from build123d import *

# Parameters (mm, degrees)
F1_DEPTH = 11.75
F3_DEPTH = 10.2
F4_R     = 3
F5_DEPTH = 12.5
F6_R     = 0.5


with BuildPart() as f1:
    # F0 (on Right) → F1 (new body, symmetric)
    with BuildSketch(Plane.YZ):
        with BuildLine():
            ThreePointArc((70.3502100474, -3.8900166392), (73.7025583371, -4.9650890437), (75.7682282921, -2.1142948795))
            ThreePointArc((75.7682282921, -2.1142948795), (73.9723491924, 0.6334483504), (70.7348330539, 0.0914484884))
            ThreePointArc((70.7348330539, 0.0914484884), (69.7821293922, -1.8258276194), (70.3502100474, -3.8900166392))
        make_face()
        with BuildLine():
            ThreePointArc((70.3502100474, -3.8900166392), (69.7821293922, -1.8258276194), (70.7348330539, 0.0914484884))
            Line((70.7348330539, 0.0914484884), (51.2349025363, 1.9752077734))
            ThreePointArc((51.2349025363, 1.9752077734), (47.3931357281, 2.2531760356), (43.5424422673, 2.3459037766))
            Line((43.5424422673, 2.3459037766), (-6.2317717079, 2.3459037766))
            Line((-6.2317717079, 2.3459037766), (-6.2317717079, -1.6540961509))
            Line((-6.2317717079, -1.6540961509), (43.5424422673, -1.6540961509))
            ThreePointArc((43.5424422673, -1.6540961509), (47.2006010586, -1.742187505), (50.8502795298, -2.0062573543))
            Line((50.8502795298, -2.0062573543), (70.3502100474, -3.8900166392))
        make_face()
    extrude(amount=F1_DEPTH, both=True)

    # F2 (on Top) → F3 (cut, symmetric)
    with BuildSketch(Plane.XY):
        with BuildLine():
            Line((8.75, 24.0882448852), (8.75, -6.2317717079))
            Line((8.75, -6.2317717079), (11.75, -6.2317717079))
            Line((11.75, -6.2317717079), (11.75, 70.7348330539))
            add(Edge.make_bspline(
                [(11.75, 70.7348330539), (11.6262901574, 67.5527974963), (11.3494589509, 59.7203740039), (8.5420361296, 34.7760059385), (8.75, 27.7926027775), (8.75, 24.0882448852)],
                knots=[0, 0, 0, 0, 0.2868478111, 0.7138684007, 1, 1, 1, 1], degree=3))
        make_face()
        with BuildLine():
            Line((-11.75, -6.2317717079), (-8.75, -6.2317717079))
            Line((-8.75, -6.2317717079), (-8.75, 24.0882448852))
            add(Edge.make_bspline(
                [(-11.75, 70.7348330539), (-11.6262901574, 67.5527974963), (-11.3494589509, 59.7203740039), (-8.5420361296, 34.7760059385), (-8.75, 27.7926027775), (-8.75, 24.0882448852)],
                knots=[0, 0, 0, 0, 0.2868478111, 0.7138684007, 1, 1, 1, 1], degree=3))
            Line((-11.75, 70.7348330539), (-11.75, -6.2317717079))
        make_face()
    extrude(amount=F3_DEPTH, both=True, mode=Mode.SUBTRACT)

    # F4 (on Right) → F5 (join, symmetric)
    with BuildSketch(Plane.YZ):
        with Locations((72.7682282921, -2.1142948795)):
            Circle(F4_R)
    extrude(amount=F5_DEPTH, both=True)

    # F6
    f6_edges = [f1.edges().sort_by_distance(p)[0] for p in [
        (12.5, 69.768228, -2.114295),
        (-12.5, 69.768228, -2.114295),
    ]]
    fillet(f6_edges, radius=F6_R)


solid = f1.part
Input: part model. Units: mm. Frame: model coordinates. A direction names the side the tool comes from. Give positions to 0.01 mm unless a question says otherwise; leave off trailing zeros. Order: outer loops, then holes, each group sorted by start corner. A loop starts at its lowest first (then second) coordinate and runs counter-clockwise, first axis right, second up. Notation, with made-up numbers: (13.25, 17) - (71.25, 17) arc R15 ccw to (71.25, 34) - close; hole circle Ø4 at (23.25, 41). An arc over 180 degrees is marked (long way). Write each question's results on one line, items separated by ' | '.
Item 1: Material intervals for line 1 along Z through (x, y) = (-8, 72.5); line 2 along Z through (x, y) = (0.25, 44); line 3 along X through (y, z) = (8, 1.5), sorted ascending.
A:
line 1: z = -5.1 to 0.87 | line 2: z = -1.66 to 2.34 | line 3: x = -8.75 to 8.75
Item 2: Access query for faces 1 (the flat face through (0, 19, 2.346)), 2 (the flat face through (8.75, 9, 0)), 3 (the flat face through (-8.75, 9, 0)). Directions: +Z, -Z, +X, -X, +Y, -Y. A direction counts if a zero-diameter tool reaches every point of the face in a straight line with its end or side. Return the directions, or none.
A:
face 1: +Z, +X, -X, +Y, -Y | face 2: +Z, -Z, +X, -Y | face 3: +Z, -Z, -X, -Y
Item 3: Section A-A (x = 4.5). Return loops of the section in (y, z), and give its area (3 significant figures).
A:
outline: (-6.23, -1.65) - (43.54, -1.65) arc R76 cw to (50.85, -2.01) - (70.35, -3.89) arc R3 ccw (long way) to (70.73, 0.09) - (51.23, 1.98) arc R80 ccw to (43.54, 2.35) - (-6.23, 2.35) - close | area: 334 mm^2
Item 4: Contact query for flat-ended pins moving along their axis: pin 1 Ø4 at (x, y) = (9, 57.5) entering from -Z; pin 2 Ø1.5 at (x, y) = (-5, 66) entering from +Z; pin 3 Ø3 at (y, z) = (16.5, -0.5) entering from +X. Output: stop coordinate, or through.
A:
pin 1: stops at z = -2.84 | pin 2: stops at z = 0.62 | pin 3: stops at x = 8.75
Item 5: Draft query along Y for faces 4 (the flat face through (0.16, 61.12, 1.02)), 5 (the flat face through (0, 18, -1.654)), 6 (the flat face through (0, -6.232, 0)). Return one class per face: released by +Y, released by -Y, zero draft, split by the parting line, or undercut.
A:
face 4: undercut | face 5: zero draft | face 6: released by -Y
Item 6: Section B-B (y = 5.5). Return loops of the section in (x, z), and give its area (3 significant figures).
A:
outline: (-8.75, -1.65) - (8.75, -1.65) - (8.75, 2.35) - (-8.75, 2.35) - close | area: 70.0 mm^2
